Source: CAD feature listing. Evaluate the final solid. Frame: model axes, mm. A direction names the side the tool comes from. Coordinates: 2 decimals unless noted, no trailing zeros. Write each loop counter-clockwise with the first axis right and the second up, starting at its lowest first coordinate (ties: lowest second). Pieces come first, ordered by that corner, then holes. Notation, with made-up numbers: M 27,26 L 39,26 A29 cw 39,49 Z; hole C 89,64 d1. An arc over 180 degrees is marked long. Write item = value, one per line. Start each with the question number.
1. Access query for faces 1 (the face through (26, 15, 3)), 2 (the face through (4.3, 12.3, 0)), 3 (the face through (0, 15, 1)). Directions: +Z, -Z, +X, -X, +Y, -Y. A direction counts if a zero-diameter tool reaches every point of the face in a straight line with its end or side. Return the directions, or none.
2. Line query: line 1 along Y through (x, z) = (0, 17); line 2 along X through (y, z) = (-30, 9.75); line 3 along X through (y, z) = (14, 6.5). Output: solid intervals per line, ascending.
3. Pull-direction query (X, two-part tool) for faces 4 (the face through (-5, 13, 3)), 5 (the face through (2, -31, 25)); classes: pulls with the +X half, pulls with the -X half, needs draft (parallel to the pull), parting line crosses it, or undercut.
4. Section query A-A (z = 20). Output: boundary loops of the cut face in (x, y) (3 decimals).
5. Pin query (flat end, axial travel): pin 1 Ø2 at (x, y) = (-25.98, 15) entering from +Z; pin 2 Ø10 at (x, z) = (-8.5, 18.5) entering from -Y; pin 3 Ø1.5 at (x, z) = (-2.5, 14.5) entering from -Y; pin 4 Ø4 at (x, y) = (0, -30.5) entering from +Z. Return the tip coordinate at first contact, or that it passes through.
```python
from build123d import *

# Parameters (mm, degrees)
F1_DEPTH = 3
F2_DEPTH = 25
F3_SIZE  = 1
F4_SIZE  = 1.99999


# Not quite as in the source:
# - a fillet or chamfer is up to 0.001 mm smaller than in the source, because OpenCascade refuses the exact size


with BuildPart() as f1:
    # F0 (on Top) → F1 (new body)
    with BuildSketch(Plane.XY):
        with BuildLine():
            ThreePointArc((-6.1694813396, 10), (0, 11.75), (6.1694813396, 10))
            Line((6.1694813396, 10), (23.0940107676, 10))
            Line((23.0940107676, 10), (23.9807621135, 11.5358983849))
            ThreePointArc((23.9807621135, 11.5358983849), (22.5166604984, 13), (21.9807621135, 15))
            Line((21.9807621135, 15), (-21.9807621135, 15))
            ThreePointArc((-21.9807621135, 15), (-22.5166604984, 13), (-23.9807621135, 11.5358983849))
            Line((-23.9807621135, 11.5358983849), (-23.0940107676, 10))
            Line((-23.0940107676, 10), (-6.1694813396, 10))
        make_face()
        with BuildLine():
            ThreePointArc((-6.1694813396, -10), (-11.75, 0), (-6.1694813396, 10))
            Line((-6.1694813396, 10), (-23.0940107676, 10))
            Line((-23.0940107676, 10), (-11.5470053838, -10))
            Line((-11.5470053838, -10), (-6.1694813396, -10))
        make_face()
        with BuildLine():
            Line((11.5470053838, -10), (6.1694813396, -10))
            ThreePointArc((6.1694813396, -10), (0, -11.75), (-6.1694813396, -10))
            Line((-6.1694813396, -10), (-11.5470053838, -10))
            Line((-11.5470053838, -10), (-2, -26.5358983849))
            ThreePointArc((-2, -26.5358983849), (0, -26), (2, -26.5358983849))
            Line((2, -26.5358983849), (11.5470053838, -10))
        make_face()
        with BuildLine():
            ThreePointArc((6.1694813396, 10), (10.2604557828, 5.725866496), (11.75, 0))
            ThreePointArc((11.75, 0), (10.2604557828, -5.725866496), (6.1694813396, -10))
            Line((6.1694813396, -10), (11.5470053838, -10))
            Line((11.5470053838, -10), (23.0940107676, 10))
            Line((23.0940107676, 10), (6.1694813396, 10))
        make_face()
    extrude(amount=F1_DEPTH)



with BuildPart() as f1b:
    # F0 (on Top) → F1, piece 2 (new body)
    with BuildSketch(Plane.XY):
        with BuildLine():
            ThreePointArc((1.75, -30), (1.5155444566, -29.125), (0.875, -28.4844555434))
            Line((0.875, -28.4844555434), (0, -30))
            Line((0, -30), (-0.875, -28.4844555434))
            ThreePointArc((-0.875, -28.4844555434), (-0.875, -31.5155444566), (1.75, -30))
        make_face()
        with BuildLine():
            Line((0, -30), (0.875, -28.4844555434))
            ThreePointArc((0.875, -28.4844555434), (0, -28.25), (-0.875, -28.4844555434))
            Line((-0.875, -28.4844555434), (0, -30))
        make_face()
    extrude(amount=F1_DEPTH)


with BuildPart() as f1c:
    # F0 (on Top) → F1, piece 3 (new body)
    with BuildSketch(Plane.XY):
        with BuildLine():
            ThreePointArc((24.2307621135, 15), (24.4652176569, 14.125), (25.1057621135, 13.4844555434))
            Line((25.1057621135, 13.4844555434), (25.9807621135, 15))
            Line((25.9807621135, 15), (24.2307621135, 15))
        make_face()
        with BuildLine():
            Line((25.9807621135, 15), (25.1057621135, 13.4844555434))
            ThreePointArc((25.1057621135, 13.4844555434), (26.8557621135, 13.4844555434), (27.7307621135, 15))
            ThreePointArc((27.7307621135, 15), (25.9807621135, 16.75), (24.2307621135, 15))
            Line((24.2307621135, 15), (25.9807621135, 15))
        make_face()
    extrude(amount=F1_DEPTH)


with BuildPart() as f1d:
    # F0 (on Top) → F1, piece 4 (new body)
    with BuildSketch(Plane.XY):
        with BuildLine():
            Line((-25.9807621135, 15), (-25.1057621135, 13.4844555434))
            ThreePointArc((-25.1057621135, 13.4844555434), (-24.4652176569, 14.125), (-24.2307621135, 15))
            Line((-24.2307621135, 15), (-25.9807621135, 15))
        make_face()
        with BuildLine():
            ThreePointArc((-24.2307621135, 15), (-27.4963065702, 15.875), (-25.1057621135, 13.4844555434))
            Line((-25.1057621135, 13.4844555434), (-25.9807621135, 15))
            Line((-25.9807621135, 15), (-24.2307621135, 15))
        make_face()
    extrude(amount=F1_DEPTH)


with BuildPart() as f1_1:
    add(f1.part)

    add(f1b.part)  # F2 merges F1b

    add(f1c.part)  # F2 merges F1c

    add(f1d.part)  # F2 merges F1d
    # F0 (on Top) → F2 (join)
    with BuildSketch(Plane.XY):
        with BuildLine():
            Line((-25.1057621135, 13.4844555434), (-23.9807621135, 11.5358983849))
            ThreePointArc((-23.9807621135, 11.5358983849), (-22.5166604984, 13), (-21.9807621135, 15))
            Line((-21.9807621135, 15), (-24.2307621135, 15))
            ThreePointArc((-24.2307621135, 15), (-24.4652176569, 14.125), (-25.1057621135, 13.4844555434))
        make_face()
        with BuildLine():
            ThreePointArc((-21.9807621135, 15), (-29.4448637287, 17), (-23.9807621135, 11.5358983849))
            Line((-23.9807621135, 11.5358983849), (-25.1057621135, 13.4844555434))
            ThreePointArc((-25.1057621135, 13.4844555434), (-27.4963065702, 15.875), (-24.2307621135, 15))
            Line((-24.2307621135, 15), (-21.9807621135, 15))
        make_face()
        with BuildLine():
            ThreePointArc((21.9807621135, 15), (22.5166604984, 13), (23.9807621135, 11.5358983849))
            Line((23.9807621135, 11.5358983849), (25.1057621135, 13.4844555434))
            ThreePointArc((25.1057621135, 13.4844555434), (24.4652176569, 14.125), (24.2307621135, 15))
            Line((24.2307621135, 15), (21.9807621135, 15))
        make_face()
        with BuildLine():
            Line((25.1057621135, 13.4844555434), (23.9807621135, 11.5358983849))
            ThreePointArc((23.9807621135, 11.5358983849), (27.9807621135, 11.5358983849), (29.9807621135, 15))
            ThreePointArc((29.9807621135, 15), (25.9807621135, 19), (21.9807621135, 15))
            Line((21.9807621135, 15), (24.2307621135, 15))
            ThreePointArc((24.2307621135, 15), (25.9807621135, 16.75), (27.7307621135, 15))
            ThreePointArc((27.7307621135, 15), (26.8557621135, 13.4844555434), (25.1057621135, 13.4844555434))
        make_face()
        with BuildLine():
            Line((0.875, -28.4844555434), (2, -26.5358983849))
            ThreePointArc((2, -26.5358983849), (0, -26), (-2, -26.5358983849))
            Line((-2, -26.5358983849), (-0.875, -28.4844555434))
            ThreePointArc((-0.875, -28.4844555434), (0, -28.25), (0.875, -28.4844555434))
        make_face()
        with BuildLine():
            ThreePointArc((4, -30), (3.4641016151, -28), (2, -26.5358983849))
            Line((2, -26.5358983849), (0.875, -28.4844555434))
            ThreePointArc((0.875, -28.4844555434), (1.5155444566, -29.125), (1.75, -30))
            ThreePointArc((1.75, -30), (-0.875, -31.5155444566), (-0.875, -28.4844555434))
            Line((-0.875, -28.4844555434), (-2, -26.5358983849))
            ThreePointArc((-2, -26.5358983849), (-2, -33.4641016151), (4, -30))
        make_face()
    extrude(amount=F2_DEPTH)

    # F3
    f3_edges = [f1_1.edges().sort_by_distance(p)[0] for p in [
        (-6.169481, -10, 0),
    ]]
    chamfer(f3_edges, length=F3_SIZE)

    # F4 (size 2 in the source; OpenCascade refuses exactly that, so slightly less here)
    f4_edges = [f1_1.edges().sort_by_distance(p)[0] for p in [
        (-6.169481, -10, 3),
    ]]
    chamfer(f4_edges, length=F4_SIZE)


solid = f1_1.part
```
Results are:
q1.face_1 = +Z
q1.face_2 = -Z, +X, -X, +Y, -Y
q1.face_3 = +Z, -Z, +Y
q2.line_1 = -34 to -31.75, -28.25 to -26
q2.line_2 = -4 to -1.75, 1.75 to 4
q2.line_3 = -29.85 to -27.42, -24.54 to -22.11, 22.11 to 24.54, 27.42 to 29.85
q3.face_4 = undercut
q3.face_5 = needs draft
q4.outline = C -25.981,15 d8; C 0,-30 d8; C 25.981,15 d8; hole C -25.981,15 d3.5; hole C 0,-30 d3.5; hole C 25.981,15 d3.5
q5.pin_1 = 3
q5.pin_2 = -31.94
q5.pin_3 = -33.6
q5.pin_4 = 25
